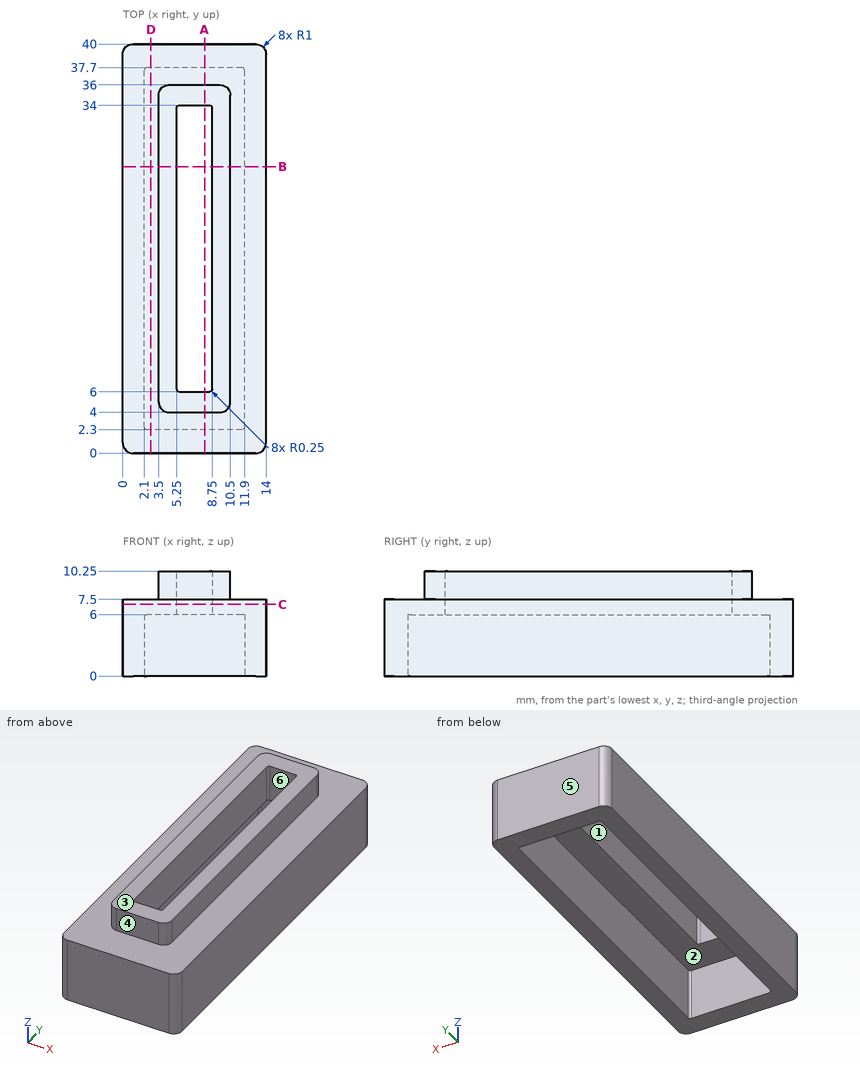
Geometry: see drawing. Coordinates: mm, zero at the bounding-box minimum. A direction names the side the tool comes from. Give positions to 0.01 mm unless a question says otherwise; leave off trailing zeros. Order: outer loops, then holes, each group sorted by start corner. A loop starts at its lowest first (then second) coordinate and runs counter-clockwise, first axis right, second up.
1. Cut plane B-B (y = 28). Return loops of the section in (x, z).
Computed:
outline: (0, 0) - (2.1, 0) - (2.1, 6) - (5.25, 6) - (5.25, 10.25) - (3.5, 10.25) - (3.5, 7.5) - (0, 7.5) - close; (8.75, 6) - (11.9, 6) - (11.9, 0) - (14, 0) - (14, 7.5) - (10.5, 7.5) - (10.5, 10.25) - (8.75, 10.25) - close
2. Set-up query: the marked faces 1, 2 and 3. Return all of +Z, -Z, +X, -X, +Y, -Y with unobstructed straight access to the full face (end or side cutting, diameter ignored); none if empty.
Computed:
face 1: +Z, -Z
face 2: -Z
face 3: +Z, +X, -X, +Y, -Y
3. Pin query (flat end, axial travel): pin 1 Ø1.5 at (x, z) = (7, 9) entering from +Y; pin 2 Ø5 at (x, y) = (8.5, 16.5) entering from -Z; pin 3 Ø0.8 at (x, z) = (7, 8.5) entering from -Y. Return the tip coordinate at first contact, or that it passes through.
Computed:
pin 1: stops at y = 36
pin 2: stops at z = 6
pin 3: stops at y = 4
4. Draft query along Y for the marked faces 4, 5 and 6. Return one class per face: released by +Y, released by -Y, zero draft, split by the parting line, or undercut.
Computed:
face 4: released by -Y
face 5: released by +Y
face 6: undercut
5. Cut plane C-C (z = 7). Return loops of the section in (x, y), and give its area (3 significant figures).
Computed:
outline: (0, 1) arc R1 ccw to (1, 0) - (13, 0) arc R1 ccw to (14, 1) - (14, 39) arc R1 ccw to (13, 40) - (1, 40) arc R1 ccw to (0, 39) - close; hole (5.25, 6.25) arc R0.25 ccw to (5.5, 6) - (8.5, 6) arc R0.25 ccw to (8.75, 6.25) - (8.75, 33.75) arc R0.25 ccw to (8.5, 34) - (5.5, 34) arc R0.25 ccw to (5.25, 33.75) - close
area: 461 mm2
6. Line query: probe 1 along X at (y, z) = (16, 4.75); probe 2 along Y at (x, z) = (2.75, 4); probe 3 along X at (y, z) = (27.5, 8.5). Output: solid intervals per line, ascending.
Computed:
probe 1: x = 0 to 2.1, 11.9 to 14
probe 2: y = 0 to 2.3, 37.7 to 40
probe 3: x = 3.5 to 5.25, 8.75 to 10.5
7. Cut plane A-A (x = 8). Return loops of the section in (y, z).
Computed:
outline: (0, 0) - (2.3, 0) - (2.3, 6) - (6, 6) - (6, 10.25) - (4, 10.25) - (4, 7.5) - (0, 7.5) - close; (34, 6) - (37.7, 6) - (37.7, 0) - (40, 0) - (40, 7.5) - (36, 7.5) - (36, 10.25) - (34, 10.25) - close
8. Cut plane D-D (x = 2.75). Return loops of the section in (y, z), and give its area (3 significant figures).
Computed:
outline: (0, 0) - (2.3, 0) - (2.3, 6) - (37.7, 6) - (37.7, 0) - (40, 0) - (40, 7.5) - (0, 7.5) - close
area: 87.6 mm2
